Verification items for this drawing (mm, ordinates from the low corner). A direction names the side the tool comes from. Round coordinates to 2 decimals unless told otherwise and drop trailing zeros. Order: outer loops, then holes, each group sorted by start corner. A loop starts at its lowest first (then second) coordinate and runs counter-clockwise, first axis right, second up. Notation, with made-up numbers: (43.5, 27.25) - (63.5, 27.25) arc R13 cw to (63.5, 43.25) - close; hole circle Ø8 at (-7.75, -32). An arc over 180 degrees is marked (long way). Return JSON: item names as keys, results as strings. Group by question number.
Q1. Tool access check on the marked faces 4, 5, 6, 7 and 8. Record the directions out of +Z, -Z, +X, -X, +Y, -Y that give a thin tool (end or side, any length) a straight path to the whole face; none if there is none.
Q2. Gauge pin test, flat ends, axial feed: pin 1 Ø25 at (x, z) = (184.5, 49) entering from -Y; pin 2 Ø7.5 at (x, y) = (123.5, 90.5) entering from +Z; pin 3 Ø6 at (x, z) = (154.5, 41.5) entering from -Y; pin 4 Ø12 at (y, z) = (89.5, 74.5) entering from -X. Record the tip position at first contact, or that the pin passes through.
Q3. Sectioned sample at A-A, the plane y = 24.5. Record the cut outline in (x, z).
Q4. Draft check along Z on the marked faces 1, 2 and 3. Enter one of: pulls with the +Z half, pulls with the -Z half, needs draft (parallel to the pull), parting line crosses it, or undercut.
Q5. Material ranges on line 1 along X through (y, z) = (54, 39); line 2 along Y through (x, z) = (38.5, 33); line 3 along Y through (x, z) = (168.5, 50.5), recorded low to high.
Q6. Sectioned sample at D-D, the plane y = 58. Record the cut outline in (x, z), then the cut area to 3 significant figures.
Q7. Sectioned sample at C-C, the plane x = 135. Record the cut outline in (y, z).
Q8. Sectioned sample at B-B, the plane z = 26. Record the cut outline in (x, y).
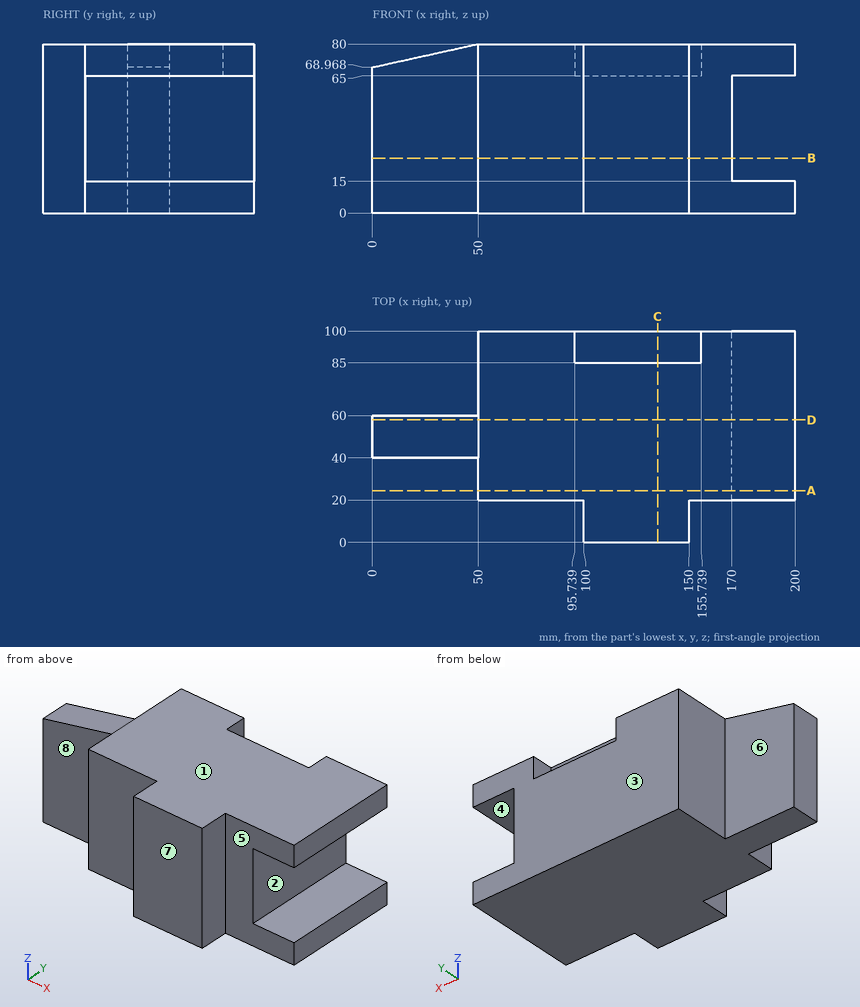
Reply:
{
 "1": {"face 4": "+X, +Y, -Y", "face 5": "+Z, -Z, +X, -Y", "face 6": "+Z, -Z, -X, +Y", "face 7": "+Z, -Z, +X, -X, -Y", "face 8": "+Z, -Z, -X, -Y"},
 "2": {"pin 1": "through", "pin 2": "z = 65", "pin 3": "y = 20", "pin 4": "x = 50"},
 "3": {"outline": "(50, 0) - (200, 0) - (200, 15) - (170, 15) - (170, 65) - (200, 65) - (200, 80) - (50, 80) - close"},
 "4": {"face 1": "pulls with the +Z half", "face 2": "undercut", "face 3": "needs draft"},
 "5": {"line 1": "0 to 170", "line 2": "40 to 60", "line 3": "20 to 100"},
 "6": {"outline": "(0, 0) - (200, 0) - (200, 15) - (170, 15) - (170, 65) - (200, 65) - (200, 80) - (50, 80) - (0, 68.97) - close", "area": "14,200 mm^2"},
 "7": {"outline": "(0, 0) - (100, 0) - (100, 65) - (85, 65) - (85, 80) - (0, 80) - close"},
 "8": {"outline": "(0, 40) - (50, 40) - (50, 20) - (100, 20) - (100, 0) - (150, 0) - (150, 20) - (170, 20) - (170, 100) - (50, 100) - (50, 60) - (0, 60) - close"}
}
